Can you work these out from the model? Positions are in its coordinate system, mm. A direction names the side the tool comes from. Coordinates: 2 decimals unless noted, no trailing zeros. Loops run counter-clockwise (first coordinate to the right, second up) from the corner with the lowest first, then second, coordinate; pieces in that order, holes last.
Autodesk Inventor part; units mm, degrees
ref_plane "РабПлоскость1" through (-8, 0, -2.95) normal (1, 0, 0) x (0, 0, -1)
ref_plane "YZ Plane" through (0, 0, 0) normal (1, 0, 0) x (0, 1, 0)
ref_plane "XZ Plane" through (0, 0, 0) normal (0, 1, 0) x (-1, 0, 0)
sketch "Эскиз1" plane through (0, 0, 0) normal (0, 1, 0) x (-1, 0, 0)
  line L0 (0, 0) -> (36, 0)
  line L1 (36, 0) -> (36, -30.3)
  line L2 (36, -30.3) -> (0, -30.3)
  line L3 (0, -30.3) -> (0, 0)
  dimension "d0" = 36
  dimension "d1" = 30.3
extrude "Выдавливание1" add sketch "Эскиз1" along normal blind 3
sketch "Эскиз2" plane through (0, 3, 0) normal (0, 1, 0) x (1, 0, 0)
  line L0 (-36, 30.3) -> (-36, 0)
  line L1 (-36, 0) -> (-36, 4.55)
  line L2 (-36, 4.55) -> (-32, 4.55)
  line L3 (-36, 0) -> (0, 0)
  line L4 (-18, 0) -> (-18, 30.3)
  line L5 (0, 30.3) -> (-36, 30.3)
  line L6 (-36, 15.15) -> (0, 15.15)
  line L7 (0, 0) -> (0, 30.3)
  point P0 (-32, 25.75)
  point P1 (-4, 4.55)
  point P2 (-4, 25.75)
  dimension "d4" = 4.55
  dimension "d48" = 4
hole "Отверстие1" at (-32, 3, -4.55) at (-32, 3, -25.75) at (-4, 3, -25.75) at (-4, 3, -4.55) direction (0, -1, 0) diameter 3.2 end through all counterbore diameter 6 counterbore depth 2.15
fillet "Сопряжение1" radius 2.95 4 edges at (0, 1.5, 0) (0, 1.5, -30.3) (-36, 1.5, -30.3) (-36, 1.5, 0)
sketch "Эскиз4" plane through (0, 0, -2.95) normal (1, 0, 0) x (0, 0, -1)
  line L0 (12.2, 0) -> (12.2, -13.5)
  circle A0 centre (12.2, -13.5) radius 18.5
  line L1 (0, 0) -> (24.4, 0)
  line L2 (0, 0) -> (0, 3)
  line L3 (0, 1.5) -> (24.4, 1.5)
  line L4 (24.4, 3) -> (24.4, 0)
  dimension "d27" = 13.5
  dimension "d38" = 37
ref_plane "РабПлоскость1" through (-8, 0, -2.95) normal (1, 0, 0) x (0, 0, -1)
extrude "Выдавливание3" cut sketch "Эскиз4" against normal blind 7 from surface at -8 contours A0 L2 L1 L4 | L4 L1 L2 A0 L3 | L3 A0
sketch "Эскиз6" plane through (0, 3, 0) normal (0, 1, 0) x (1, 0, 0)
  line L0 (-15, 23.5166) -> (-15, 6.7834)
  line L1 (-15, 15.15) -> (-19.7, 15.15)
  line L2 (-19.7, 6.25) -> (-19.7, 24.05)
  point P0 (0, 0)
  dimension "d39" = 4.7
  dimension "d40" = 17.8
hole "Отверстие2" at (-19.7, 3, -6.25) at (-19.7, 3, -24.05) direction (0, -1, 0) diameter 2.2 end through all
sketch "Эскиз7" plane through (0, 0, 0) normal (0, -1, 0) x (1, 0, 0)
  circle A0 centre (-19.7, -6.25) radius 1.1
  line L0 (-17.35, -7.6068) -> (-19.7, -8.9635)
  line L1 (-19.7, -8.9635) -> (-22.05, -7.6068)
  line L2 (-22.05, -7.6068) -> (-22.05, -4.8932)
  line L3 (-22.05, -4.8932) -> (-19.7, -3.5365)
  line L4 (-19.7, -3.5365) -> (-17.35, -4.8932)
  line L5 (-17.35, -4.8932) -> (-17.35, -7.6068)
  circle A1 centre (-19.7, -24.05) radius 1.1
  line L6 (-17.35, -25.4068) -> (-19.7, -26.7635)
  line L7 (-19.7, -26.7635) -> (-22.05, -25.4068)
  line L8 (-22.05, -25.4068) -> (-22.05, -22.6932)
  line L9 (-22.05, -22.6932) -> (-19.7, -21.3365)
  line L10 (-19.7, -21.3365) -> (-17.35, -22.6932)
  line L11 (-17.35, -22.6932) -> (-17.35, -25.4068)
  line L12 (-15, -2.5009) -> (-15, -27.7991)
  point P0 (0, 0)
  dimension "d49" = 4.7
extrude "Выдавливание4" cut sketch "Эскиз7" against normal blind 2.1
equation "\"Радиус_гибки\" = Толщина"
equation "\"Ширина_просечки\" = Толщина"
equation "\"Глубина_просечки\" = 0.5 * Толщина"
equation "\"Размер_просечки\" = 4 * Толщина"
equation "\"Мин_остаток\" = 2 * Толщина"
equation "\"Радиус_перехода\" = Радиус_гибки"
equation "\"Радиус_Якоби\" = Толщина"
equation "\"Размер_зазора\" = Толщина"
properties part number "Крепление двигателя2"
(1) I want a section at B-B on x = -4. Write out the boundary of the cut face in (y, z), then the cut area to 3 significant figures.
Check values:
outline: (0, -30.3) - (3, -30.3) - (3, -28.75) - (0.85, -28.75) - (0.85, -27.35) - (0, -27.35) - close; (0, -24.15) - (0.85, -24.15) - (0.85, -22.75) - (3, -22.75) - (3, -7.55) - (0.85, -7.55) - (0.85, -6.15) - (0, -6.15) - close; (0, -2.95) - (0.85, -2.95) - (0.85, -1.55) - (3, -1.55) - (3, 0) - (0, 0) - close
area: 59.7 mm2
(2) I want a section at A-A on z = -18. Write out the boundary of the cut face in (x, y), then the cut area to 3 significant figures.
Check values:
outline: (-36, 0) - (-15, 0) - (-15, 3) - (-36, 3) - close; (-8, 0) - (0, 0) - (0, 3) - (-8, 3) - close
area: 87.0 mm2
(3) I want a section at C-C on y = 2.5. Write out the boundary of the cut face in (x, z), then the cut area to 3 significant figures.
Check values:
outline: (-36, -27.35) arc R2.95 ccw to (-33.05, -30.3) - (-2.95, -30.3) arc R2.95 ccw to (0, -27.35) - (0, -2.95) arc R2.95 ccw to (-2.95, 0) - (-33.05, 0) arc R2.95 ccw to (-36, -2.95) - close; hole circle Ø6 at (-32, -25.75); hole circle Ø6 at (-32, -4.55); hole circle Ø2.2 at (-19.7, -24.05); hole circle Ø2.2 at (-19.7, -6.25); hole (-15, -24.44) - (-8, -24.44) - (-8, -5.86) - (-15, -5.86) - close; hole circle Ø6 at (-4, -25.75); hole circle Ø6 at (-4, -4.55)
area: 833 mm2
(4) I'm going to push flat-ended pins straight in: pin 1 (1.5 mm diameter, centred on x = -3.5, z = -10, fed in from -Y); pin 2 (1.8 mm diameter, centred on x = -30.5, z = -4.5, fed in from +Y); pin 3 (2 mm diameter, centred on x = -19.7, z = -24.05, fed in from -Y); pin 4 (2.5 mm diameter, centred on x = -19.7, z = -6.25, fed in from -Y). Where does each tip first touch, or does it pass through?
Check values:
pin 1: stops at y = 0
pin 2: stops at y = 0.85
pin 3: passes through
pin 4: stops at y = 2.1
(5) If I drill on probe 1 along Z at (x, y) = (-32, 0.65); probe 2 along X at (y, z) = (2.25, -25.75); probe 3 along Z at (x, y) = (-4, 2.25), over which ranges is the centre line in solid material (lowest first)?
Check values:
probe 1: z = -30.3 to -27.35, -24.15 to -6.15, -2.95 to 0
probe 2: x = -36 to -35, -29 to -7, -1 to 0
probe 3: z = -30.3 to -28.75, -22.75 to -7.55, -1.55 to 0
(6) If we mould it in two halves opening along Z, with no side actions, what happens to faces 4 (the cylindrical face through (-0.84, 1.52, -29.41)), 5 (the flat face through (-18, 0, -15)), 6 (the cylindrical face through (-32.132, 1.91, -28.747)), 7 (the cylindrical face through (-35.16, 1.52, -0.89))? For each: released by +Z, released by -Z, zero draft, split by the parting line, or undercut.
Check values:
face 4: released by -Z
face 5: zero draft
face 6: undercut
face 7: released by +Z
(7) I want a section at D-D on x = -34. Write out the boundary of the cut face in (y, z), then the cut area to 3 significant figures.
Check values:
outline: (0, -30.14) - (3, -30.14) - (3, -27.99) - (0.85, -27.99) - (0.85, -23.51) - (3, -23.51) - (3, -6.79) - (0.85, -6.79) - (0.85, -2.31) - (3, -2.31) - (3, -0.16) - (0, -0.16) - close
area: 70.7 mm2
(8) Which directions (+Z, -Z, +X, -X, +Y, -Y) give clear straight access to the entire face, cutting with the end or side of a thin tool? Please do faces 1 (the flat face through (-18, 3, -15)), 2 (the cylindrical face through (-30.85, 1.91, -1.78)), 3 (the flat face through (-20.859, 1.035, -26.095)).
Check values:
face 1: +Z, -Z, +X, -X, +Y
face 2: +Y
face 3: -Y
